```python
from build123d import *

# Parameters (mm, degrees)
F0_W     = 60
F0_H     = 250
F1_DEPTH = 125
F2_W     = 180
F2_H     = 180
F3_DEPTH = 30
F4_W     = 180
F4_H     = 120
F5_DEPTH = 30.001


with BuildPart() as f1:
    # F0 (on Right) → F1 (new body, symmetric)
    with BuildSketch(Plane.YZ):
        Rectangle(F0_W, F0_H)
    extrude(amount=F1_DEPTH, both=True)

    # F2 (on face) → F3 (cut)
    with BuildSketch(Plane.XZ.offset(30)):
        Rectangle(F2_W, F2_H)
    extrude(amount=-F3_DEPTH, mode=Mode.SUBTRACT)

    # F4 (on face) → F5 (cut, through all)
    with BuildSketch(Plane.XZ):
        Rectangle(F4_W, F4_H)
    extrude(amount=-F5_DEPTH, mode=Mode.SUBTRACT)


solid = f1.part
```
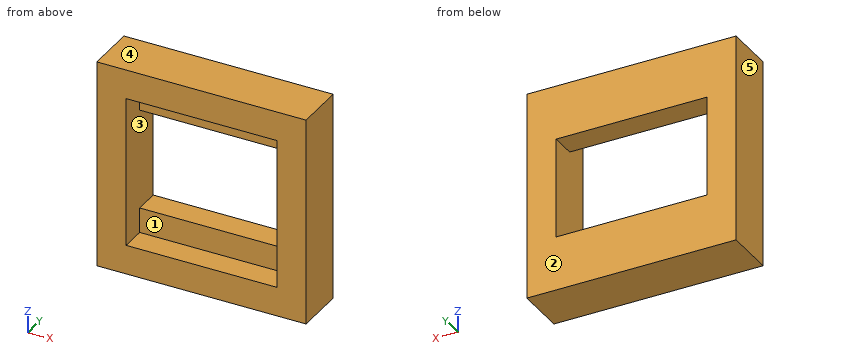
Model file for the job. Use its own axes, mm. Face numbers are marked on the shaded views. A direction names the side the tool comes from. Coordinates: 2 decimals unless noted, no trailing zeros. Write each loop counter-clockwise with the first axis right and the second up, starting at its lowest first coordinate (ties: lowest second). Pieces come first, ordered by that corner, then holes. Notation, with made-up numbers: (6.25, 23.5) - (63.25, 23.5) arc R33 cw to (63.25, 58.5) - close; hole circle Ø10 at (49, -28.5). An arc over 180 degrees is marked (long way). Use a Markdown table: item, result. Add a question column.
Item 1: Two-plate mould, pull along X, no slides. Class the marked faces 3, 4 and 5: pulls with the +X half, pulls with the -X half, needs draft (parallel to the pull), parting line crosses it, or undercut.
Item 2: Drop a flat-ended pin along its axis: pin 1 (15 mm diameter, centred on x = -36.5, z = -80.5, fed in from -Y). Give the stop position or say it passes through.
Item 3: Band-saw the part on D-D, the plane z = 72.5. Write the cut outline in (x, y).
Item 4: 3-axis set-ups, long thin cutter, end or side, ignore diameter. For the marked faces 1 and 2: which of +Z, -Z, +X, -X, +Y, -Y reach the whole face in a straight line?
Item 5: Band-saw the part on A-A, the plane z = 27. Write the cut outline in (x, y), and give its area (3 significant figures).
Item 6: Drill centre lines: line 1 along Z through (x, y) = (86.5, -11.5); line 2 along Z through (x, y) = (-35.5, 18.5). Where is each one in solid material? Low to high.
Item 7: Band-saw the part on B-B, the plane x = 63. Write the cut outline in (y, z).
Item 8: Band-saw the part on C-C, the plane y = -5. Write the cut outline in (x, z), and give its area (3 significant figures).
A:
| question | item | result |
|---|---|---|
| 1 | face 3 | undercut |
| 1 | face 4 | needs draft |
| 1 | face 5 | pulls with the -X half |
| 2 | pin 1 | stops at y = 0 |
| 3 | outline | (-125, -30) - (-90, -30) - (-90, 0) - (90, 0) - (90, -30) - (125, -30) - (125, 30) - (-125, 30) - close |
| 4 | face 1 | -Y |
| 4 | face 2 | +Z, -Z, +X, -X, +Y |
| 5 | outline | (-125, -30) - (-90, -30) - (-90, 30) - (-125, 30) - close; (90, -30) - (125, -30) - (125, 30) - (90, 30) - close |
| 5 | area | 4,200 mm² |
| 6 | line 1 | z = -125 to -90, 90 to 125 |
| 6 | line 2 | z = -125 to -60, 60 to 125 |
| 7 | outline | (-30, -125) - (30, -125) - (30, -60) - (0, -60) - (0, -90) - (-30, -90) - close; (-30, 90) - (0, 90) - (0, 60) - (30, 60) - (30, 125) - (-30, 125) - close |
| 8 | outline | (-125, -125) - (125, -125) - (125, 125) - (-125, 125) - close; hole (-90, -90) - (90, -90) - (90, 90) - (-90, 90) - close |
| 8 | area | 30,100 mm² |
